Job drawing, mm, ordinate dimensions from the low corner. One solid piece. Give positions to 0.01 mm unless a question says otherwise; leave off trailing zeros. Order: outer loops, then holes, each group sorted by start corner. A loop starts at its lowest first (then second) coordinate and runs counter-clockwise, first axis right, second up. Notation, with made-up numbers: M 42.5,42 L 88.5,42 A9 ccw 88.5,52 Z; hole C 11,-30 d9. An arc over 180 degrees is marked long. Put each result on its own line as item: value. Start each with the question number.
1) Cut at B-B (x = 2.75). Write the cut outline in (y, z) (1 decimal).
2) Cut at A-A (z = 18.5). Write the cut outline in (x, y), and give its area (3 significant figures).
3) Drill centre lines: line 1 (Z direction, x = 10.25, y = 10); line 2 (Z direction, x = 5, y = 11.5); line 3 (Y direction, x = 8.25, z = 7.5). Where is each one in solid material? Low to high. Write a range as [from, to].
4) Cut at C-C (y = 19). Write the cut outline in (x, z), and give its area (3 significant figures).
5) Pin check, flat tips, straight feed: pin 1 (6 mm diameter, centred on x = 3.5, y = 4.5, fed in from -Z); pin 2 (1 mm diameter, centred on x = 7, z = 16.5, fed in from +Y) (1 decimal); pin 3 (1 mm diameter, centred on x = 6.5, y = 11, fed in from +Z). Stop position of each tip, or through.
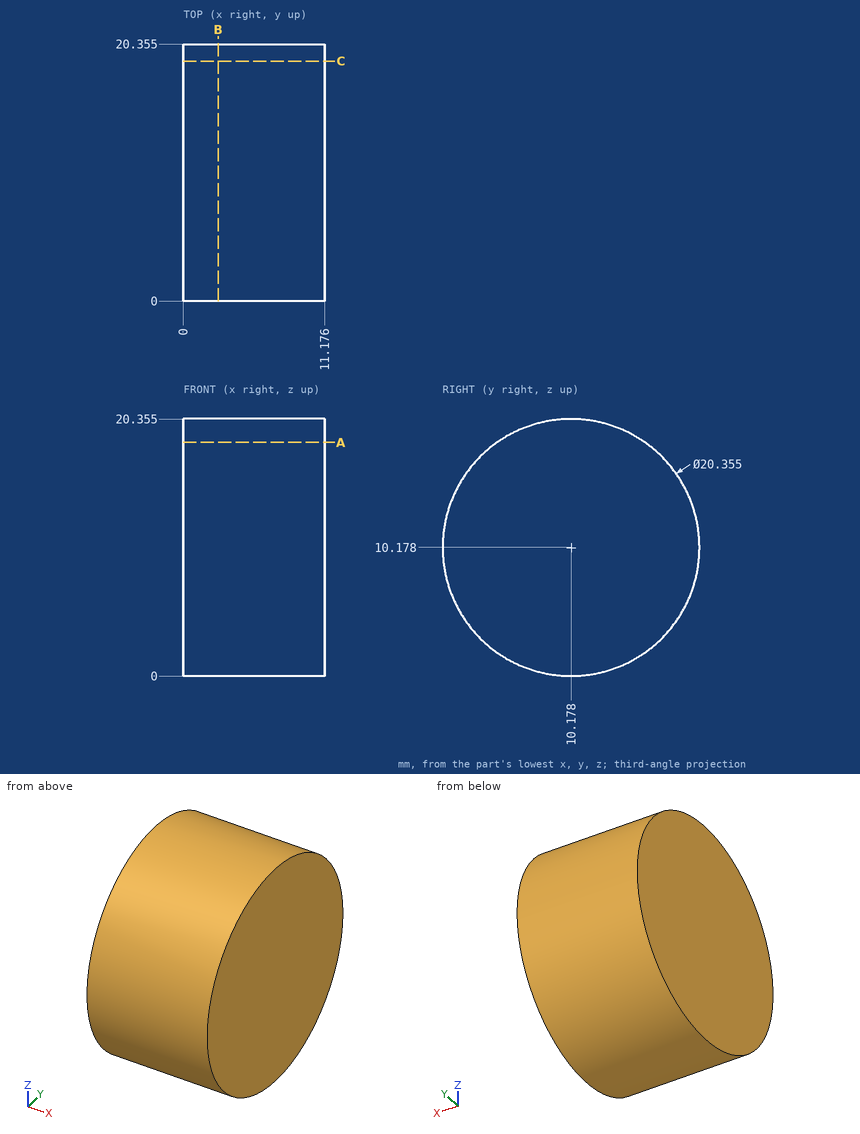
Solution:
1. outline: C 10.2,10.2 d20.4
2. outline: M 0,4.32 L 11.18,4.32 L 11.18,16.04 L 0,16.04 Z
2. area: 131 mm²
3. line 1: [0, 20.35]
3. line 2: [0.09, 20.27]
3. line 3: [0.36, 20]
4. outline: M 0,5.1 L 11.18,5.1 L 11.18,15.25 L 0,15.25 Z
4. area: 113 mm²
5. pin 1: z = 0.36
5. pin 2: y = 18.5
5. pin 3: z = 20.35
